Could you check a few things on this drawing? It's one solid part, dimensions in mm from its lowest x, y, z. A direction names the side the tool comes from. Give positions to 0.01 mm unless a question says otherwise; leave off trailing zeros. Order: outer loops, then holes, each group sorted by start corner. A loop starts at its lowest first (then second) coordinate and runs counter-clockwise, first axis right, second up. Notation, with made-up numbers: (-18, 76.5) - (19, 76.5) arc R24 ccw to (19, 99.5) - close; hole circle Ø8 at (-15, 79). An arc over 180 degrees is marked (long way). Answer as CSV lines item,"result".
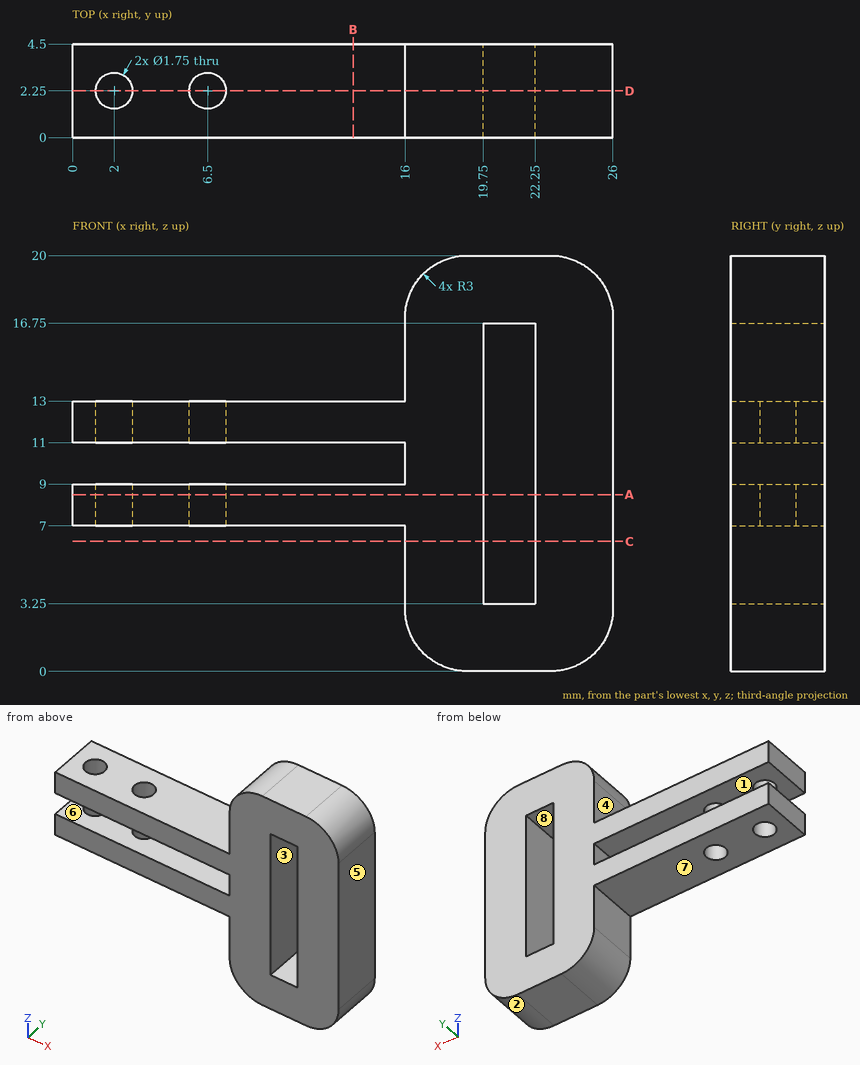
1) I'm going to push flat-ended pins straight in: P1, Ø2, axis at x = 6.5, y = 2.25, coming from the -Z side; P2, Ø1.5, axis at y = 0.5, z = 18, coming from the +X side; P3, Ø1.2, axis at y = 1.5, z = 14.5, coming from the -X side. Where does each tip first touch, or does it pass through?
Answer block:
P1,"z = 7"
P2,"x = 25.99"
P3,"x = 16"
2) If we mould it in two halves opening along X, with no side actions, what happens to the marked faces 1, 2 and 3? For each: +X half, -X half, draft (parallel to the pull), parting line (faces both ways), or undercut.
Answer block:
face 1,"draft"
face 2,"+X half"
face 3,"undercut"
3) I want a section at B-B on x = 13.5. Write out the boundary of the cut face in (y, z), plus the area to 3 significant figures.
Answer block:
outline,"(0, 7) - (4.5, 7) - (4.5, 9) - (0, 9) - close; (0, 11) - (4.5, 11) - (4.5, 13) - (0, 13) - close"
area,"18.0 mm2"
4) Which directions (+Z, -Z, +X, -X, +Y, -Y) give clear straight access to the entire face, cutting with the end or side of a thin tool? Please do the marked faces 4, 5, 6, 7 and 8.
Answer block:
face 4,"+Z, -X, +Y, -Y"
face 5,"+Z, -Z, +X, +Y, -Y"
face 6,"-X, +Y, -Y"
face 7,"-Z, -X, +Y, -Y"
face 8,"+Y, -Y"
5) I want a section at A-A on z = 8.5. Write out the boundary of the cut face in (x, y) (3 decimals).
Answer block:
outline,"(0, 0) - (19.75, 0) - (19.75, 4.5) - (0, 4.5) - close; (22.25, 0) - (26, 0) - (26, 4.5) - (22.25, 4.5) - close; hole circle Ø1.75 at (2, 2.25); hole circle Ø1.75 at (6.5, 2.25)"
6) I need wall thicknesses on line 1 along X through (y, z) = (1.9, 6.5); line 2 along Z through (x, y) = (7, 3.85); line 3 along Y through (x, z) = (2, 8.25) (3 decimals). Which ranges of each line are inside material? Lowest first, please. Write a range as [from, to].
Answer block:
line 1,"[16, 19.75], [22.25, 26]"
line 2,"[7, 9], [11, 13]"
line 3,"[0, 1.375], [3.125, 4.5]"
7) I want a section at C-C on z = 6.25. Write out the boundary of the cut face in (x, y), plus the area to 4 significant figures.
Answer block:
outline,"(16, 0) - (19.75, 0) - (19.75, 4.5) - (16, 4.5) - close; (22.25, 0) - (26, 0) - (26, 4.5) - (22.25, 4.5) - close"
area,"33.75 mm2"
8) I want a section at D-D on y = 2.25. Count the separate pieces of the cut face and the enclosed holes in it, plus the area to 3 significant figures.
Answer block:
separate pieces,"5"
enclosed holes,"1"
area,"209 mm2"
